Check sheet for the modelled part. Datum: model origin and axes. Units: mm. A direction names the side the tool comes from. Round coordinates to 2 decimals unless told otherwise and drop trailing zeros. Loops run counter-clockwise (first coordinate to the right, second up) from the corner with the lowest first, then second, coordinate; pieces in that order, holes last. Notation, with made-up numbers: M -11.75,-23.75 L -0.75,-23.75 A21 ccw -0.75,-1.75 Z; hole C 53.5,44 d9. An arc over 180 degrees is marked long. Write item = value, one per line. Start each with the question number.
(1) Set-up check for faces 1 (the face through (-43.75, 0, 4)), 2 (the face through (42.75, 0, 1)), 3 (the face through (-4, -29, 0)): record each of +Z, -Z, +X, -X, +Y, -Y from which the full face is reachable in a straight line by a thin tool's end or side.
(2) Scan lines: L1, parallel to X at y = -19, z = 1.75; L2, parallel to X at y = 22.5, z = 4.25; L3, parallel to Y at x = -18, z = 3.8. Record each from-to range of solid material in increasing order. Write a range as from..to.
(3) Cross-section at A-A on x = -19. Record the boundary of the cut face in (y, z), plus the area to 3 significant figures.
(4) Mould release check, pull along Y, two halves, no side actions. Record for faces 4 (the face through (44.9, 29.93, 2.28)), 5 (the face through (-13.7, -29.2, 4.5)), 6 (the face through (-1, -29, 4)): pulls with the +Y half, pulls with the -Y half, needs draft (parallel to the pull), parting line crosses it, or undercut.
(5) Cross-section at B-B on y = -3. Record the boundary of the cut face in (x, z), plus the area to 4 significant figures.
(6) Cross-section at C-C on z = 0.7. Record the boundary of the cut face in (x, y).
from build123d import *

# Parameters (mm, degrees)
SKETCH1_W           = 91
SKETCH1_H           = 61
BOSS_EXTRUDE1_DEPTH = 4.5
SKETCH2_W           = 87.5
SKETCH2_H           = 58
CUT_EXTRUDE1_DEPTH  = 2
SKETCH3_W           = 85.5
SKETCH3_H           = 56
CUT_EXTRUDE2_DEPTH  = 3.5
FILLET1_R           = 2


with BuildPart() as part:
    # Sketch1 → Boss-Extrude1 (new body)
    with BuildSketch(Plane.XY):
        Rectangle(SKETCH1_W, SKETCH1_H)
    extrude(amount=BOSS_EXTRUDE1_DEPTH)

    # Sketch2 → Cut-Extrude1 (cut)
    with BuildSketch(Plane.XY.offset(4.5)):
        Rectangle(SKETCH2_W, SKETCH2_H)
    extrude(amount=-CUT_EXTRUDE1_DEPTH, mode=Mode.SUBTRACT)

    # Sketch3 → Cut-Extrude2 (cut, through all)
    with BuildSketch(Plane.XY.offset(2.5)):
        Rectangle(SKETCH3_W, SKETCH3_H)
    extrude(amount=-CUT_EXTRUDE2_DEPTH, mode=Mode.SUBTRACT)

    # Fillet1
    fillet1_edges = [part.edges().sort_by_distance(p)[0] for p in [
        (45.5, -30.5, 2.25),
        (-45.5, -30.5, 2.25),
        (-45.5, 30.5, 2.25),
        (45.5, 30.5, 2.25),
    ]]
    fillet(fillet1_edges, radius=FILLET1_R)


solid = part.part
Result:
q1.face_1 = +Z
q1.face_2 = +Z, -Z
q1.face_3 = -Z, +X, -X, +Y, -Y
q2.L1 = -45.5..-42.75, 42.75..45.5
q2.L2 = -45.5..-43.75, 43.75..45.5
q2.L3 = -30.5..-29, 29..30.5
q3.outline = M -30.5,0 L -28,0 L -28,2.5 L -29,2.5 L -29,4.5 L -30.5,4.5 Z; M 28,0 L 30.5,0 L 30.5,4.5 L 29,4.5 L 29,2.5 L 28,2.5 Z
q3.area = 18.5 mm^2
q4.face_4 = pulls with the +Y half
q4.face_5 = needs draft
q4.face_6 = undercut
q5.outline = M -45.5,0 L -42.75,0 L -42.75,2.5 L -43.75,2.5 L -43.75,4.5 L -45.5,4.5 Z; M 42.75,0 L 45.5,0 L 45.5,4.5 L 43.75,4.5 L 43.75,2.5 L 42.75,2.5 Z
q5.area = 20.75 mm^2
q6.outline = M -45.5,-28.5 A2 ccw -43.5,-30.5 L 43.5,-30.5 A2 ccw 45.5,-28.5 L 45.5,28.5 A2 ccw 43.5,30.5 L -43.5,30.5 A2 ccw -45.5,28.5 Z; hole M -42.75,-28 L 42.75,-28 L 42.75,28 L -42.75,28 Z
